Part model, mm, in its own coordinate system. A direction names the side the tool comes from. Give positions to 0.01 mm unless a question says otherwise; leave off trailing zeros. Order: outer loops, then holes, each group sorted by start corner. A loop starts at its lowest first (then second) coordinate and runs counter-clockwise, first axis right, second up.
1. Slice it at B-B on y = 0. List the corners of the cut face in (x, z) (3 decimals).
2. Slice it at A-A on x = 0. List the corners of the cut face in (y, z) (3 decimals).
3. Mould opens along Y. For faces 1 (the flat face through (-1, 1, 0)), 2 (the cylindrical face through (-39.78, 36.48, 128.35)), 3 (the flat face through (0, 25.4, -27)), 4 (the cylindrical face through (-0.628, 19.139, -69.843)) say: +Y half, -Y half, draft (parallel to the pull), parting line (faces both ways), or undercut.
4. Probe line 1 (X direction, y = 1, z = 51); line 2 (Y direction, x = -21, z = -33); line 3 (Z direction, x = -7.5, y = -0.5). List the from-to ranges inside material, lowest first.
5. Slice it at C-C on x = -16. List the corners of the cut face in (y, z).
6. Slice it at D-D on z = 36.5. List the corners of the cut face in (x, y) (3 decimals), and give its area (3 significant figures).
7. Which spindle directions (+Z, -Z, +X, -X, +Y, -Y) get a long thin tool onto all of the face, cutting with end or side? Do faces 5 (the flat face through (0, -25.4, -27)), 6 (the flat face through (-28.575, 19, -21)), 7 (the flat face through (28.575, -19, -21)). Say none if no direction does.
8. Drop flat-ended pins along their axis: pin 1 Ø4 at (y, z) = (19.5, -28.5) entering from +X (3 decimals); pin 2 Ø12 at (x, z) = (26.5, 58) entering from -Y; pin 3 Ø5 at (y, z) = (18.5, 61) entering from -X. Give the stop position or say it passes through.
from build123d import *

# Parameters (mm, degrees)
SKETCH1_R          = 53.975
EXTRUDE1_DEPTH     = 260.35
SKETCH2_W          = 12.7
SKETCH2_H          = 69.85
EXTRUDE2_DEPTH     = 28.575
SKETCH3_R          = 12.7
CUT_EXTRUDE1_DEPTH = 278.481195309


with BuildPart() as part:
    # Sketch1 → Extrude1 (new body)
    with BuildSketch(Plane.XY):
        Circle(SKETCH1_R)
    extrude(amount=EXTRUDE1_DEPTH)

    # Sketch2 → Extrude2 (add, symmetric)
    with BuildSketch(Plane(origin=(0, 0, 0), x_dir=(0, -1, 0), z_dir=(1, 0, 0))):
        with Locations((-19.05, 34.925)):
            Rectangle(SKETCH2_W, SKETCH2_H)
        with Locations((19.05, 34.925)):
            Rectangle(SKETCH2_W, SKETCH2_H)
    extrude(amount=EXTRUDE2_DEPTH, both=True)

    # Sketch3 → Cut-Extrude1 (cut, through all)
    with BuildSketch(Plane(origin=(0, 25.4, 0), x_dir=(-1, 0, 0), z_dir=(0, 1, 0))):
        with Locations(Location((0, -41.275, 0), (0, 0, 90))):
            Circle(SKETCH3_R)
        with BuildLine():
            Line((-28.575, -41.275), (-28.575, -85.725))
            Line((-28.575, -85.725), (28.575, -85.725))
            Line((28.575, -85.725), (28.575, -41.275))
            ThreePointArc((28.575, -41.275), (0, -69.85), (-28.575, -41.275))
        make_face()
    extrude(amount=-CUT_EXTRUDE1_DEPTH, mode=Mode.SUBTRACT)


solid = part.part
Data:
1. outline: (-53.975, 0) - (53.975, 0) - (53.975, 260.35) - (-53.975, 260.35) - close
2. outline: (-53.975, 0) - (-25.4, 0) - (-25.4, -28.575) - (-12.7, -28.575) - (-12.7, 0) - (12.7, 0) - (12.7, -28.575) - (25.4, -28.575) - (25.4, 0) - (53.975, 0) - (53.975, 260.35) - (-53.975, 260.35) - close; (-25.4, -69.85) - (-12.7, -69.85) - (-12.7, -53.975) - (-25.4, -53.975) - close; (12.7, -69.85) - (25.4, -69.85) - (25.4, -53.975) - (12.7, -53.975) - close
3. face 1: undercut
3. face 2: parting line
3. face 3: +Y half
3. face 4: draft
4. line 1: x = -53.97 to 53.97
4. line 2: y = -25.4 to -12.7, 12.7 to 25.4
4. line 3: z = 0 to 260.35
5. outline: (-51.55, 0) - (-25.4, 0) - (-25.4, -64.95) - (-12.7, -64.95) - (-12.7, 0) - (12.7, 0) - (12.7, -64.95) - (25.4, -64.95) - (25.4, 0) - (51.55, 0) - (51.55, 260.35) - (-51.55, 260.35) - close
6. outline: circle Ø107.95 at (0, 0)
6. area: 9,150 mm2
7. face 5: -Z, +X, -X, -Y
7. face 6: -Z, -X, +Y, -Y
7. face 7: -Z, +X, +Y, -Y
8. pin 1: stops at x = 28.575
8. pin 2: stops at y = -49.93
8. pin 3: stops at x = -51.55
